CAD build for the part. Positions are in the model's coordinates, mm. Face numbers are marked on the shaded views. A direction names the side the tool comes from. Give positions to 0.01 mm unless a question says otherwise; leave off trailing zeros. Write each loop counter-clockwise with the first axis right and the second up, starting at its lowest first coordinate (ties: lowest second). Pieces come first, ordered by that corner, then holes. Notation, with made-up numbers: M 82,1 L 93,1 A13 cw 93,19 Z; hole C -30,79 d8. An arc over 180 degrees is marked long. One line per question, with ' | ' between items. Start each with the question number.
1. Cut at C-C, the plane x = 28.95. Write the cut outline in (y, z), then the cut area to 3 significant figures.
2. Cut at A-A, the plane z = 3. Count the separate pieces of the cut face and the enclosed holes in it, then the cut area to 3 significant figures.
3. Cut at B-B, the plane y = -40. Write the cut outline in (x, z) (3 decimals), then the cut area to 3 significant figures.
4. Flat gauge pin, fed straight in: pin 1 (3 mm diameter, centred on x = 16.425, y = -40, fed in from -Z). Where does the tip first touch, or does it go through?
5. Pull direction Y, two halves, no side cores. Call the marked faces 1, 2 and 3: released by +Y, released by -Y, zero draft, split by the parting line, or undercut.
6. Wall check: L1, parallel to X at y = -40, z = 4.75 (3 decimals); L2, parallel to X at y = -40, z = 3 (3 decimals); L3, parallel to X at y = -44, z = 3. Give the ranges that are in metal, low to high.
7. Which spindle directions (+Z, -Z, +X, -X, +Y, -Y) get a long thin tool onto all of the face, cutting with end or side? Do the marked faces 4 and 5. Say none if no direction does.
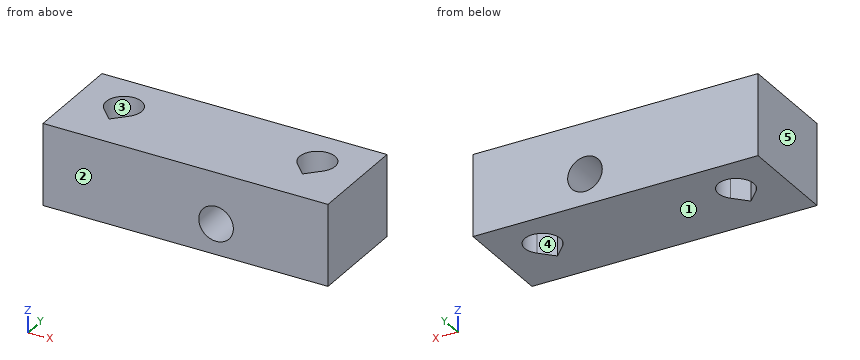
Solid Edge part; units mm, degrees
sketch "Sketch1" plane through (0, 0, 0) normal (0, 0, 1) x (1, 0, 0)
  circle A0 centre (35.425, -40) radius 1.75
  line L0 (11.95, -46) -> (39.95, -46)
  line L1 (39.95, -46) -> (39.95, -36)
  line L2 (11.95, -36) -> (39.95, -36)
  line L3 (11.95, -36) -> (11.95, -46)
  circle A1 centre (16.425, -40) radius 1.75
extrude "Protrusion1" add sketch "Sketch1" along normal blind 8
sketch "Sketch2" plane through (25.95, -46, 4) normal (0, -1, 0) x (-1, 0, 0)
  circle A0 centre (-3, 1) radius 1.7
  dimension "D1" = 3
extrude "Cutout1" cut sketch "Sketch2" against normal through all
sketch "Sketch3" plane through (25.95, -41, 8) normal (0, 0, 1) x (-1, 0, 0)
  line L0 (-9.475, -1) -> (-8.2162, 0.2157)
  line L1 (-8.2162, 0.2157) -> (-9.475, 1.5192)
  line L2 (-9.475, 1.5192) -> (-10.7338, 0.2157)
  line L3 (-10.7338, 0.2157) -> (-9.475, -1)
  line L4 (9.525, -1) -> (10.7838, 0.2157)
  line L5 (10.7838, 0.2157) -> (9.525, 1.5192)
  line L6 (9.525, 1.5192) -> (8.2662, 0.2157)
  line L7 (8.2662, 0.2157) -> (9.525, -1)
extrude "Cutout2" cut sketch "Sketch3" against normal through all
Here are the results:
1) outline: M -46,0 L -36,0 L -36,1.3 L -46,1.3 Z; M -46,4.7 L -36,4.7 L -36,8 L -46,8 Z | area: 46.0 mm^2
2) separate pieces: 2 | enclosed holes: 2 | area: 225 mm^2
3) outline: M 11.95,0 L 14.675,0 L 14.675,8 L 11.95,8 Z; M 18.175,0 L 33.675,0 L 33.675,8 L 18.175,8 Z; M 37.175,0 L 39.95,0 L 39.95,8 L 37.175,8 Z; hole C 28.95,3 d3.4 | area: 159 mm^2
4) pin 1: through
5) face 1: zero draft | face 2: released by -Y | face 3: undercut
6) L1: 11.95 to 14.675, 18.175 to 33.675, 37.175 to 39.95 | L2: 11.95 to 14.675, 18.175 to 27.25, 30.65 to 33.675, 37.175 to 39.95 | L3: 11.95 to 27.25, 30.65 to 39.95
7) face 4: +Z, -Z | face 5: +Z, -Z, -X, +Y, -Y
